Read the model definition and answer for the solid it produces. Units are mm, in the model's axes. A direction names the side the tool comes from. Coordinates: 2 decimals unless noted, no trailing zeros. Write each loop counter-clockwise with the first axis right and the second up, starting at its lowest first coordinate (ties: lowest second). Pieces come first, ordered by that corner, then holes. Notation, with made-up numbers: (82.25, 52.25) -> (141.25, 52.25) arc R19 cw to (141.25, 61.25) -> close; hole circle Ø5 at (-19.5, -16.5). An arc over 180 degrees is marked (long way). Answer as a JSON object with one key per item and string values. Group by question number.
(1) Find section C-C (x = 46). Give the vertices of the cut face in (y, z).
(2) For a pull along X with two mould halves and no side action, classify faces 4 (the face through (98.32, 3.24, 1.48)), 5 (the face through (97.908, -0.601, 1.479)), 6 (the face through (-94.092, -0.601, 1.479)), 7 (the face through (-3, 0, 6)) as +X half, -X half, draft (parallel to the pull), parting line (faces both ways), or undercut.
(3) Flat-ended cylindrical pins translate along their axes: P1, Ø2.5, axis at x = -44.5, y = 0, coming from the +Z side; P2, Ø4, axis at y = 2.5, z = -6, coming from the -X side; P3, Ø10, axis at x = 3.5, z = 6.5, coming from the -Y side; P4, Ø3, axis at y = -2, z = 3.5, coming from the -X side. Find the tip coordinate at first contact, or state that the pin passes through.
(4) Straight lines are drawn through the part: L1, parallel to Z at x = 88, y = 4.25; L2, parallel to Y at x = -96, z = 1.55; L3, parallel to X at y = -1.5, z = 8.5. For each, find the intervals that lie inside material, in ascending order.
(5) Find section A-A (x = 0). Give the vertices of the cut face in (y, z).
(6) Find section B-B (z = -3.5). Give the vertices of the cut face in (x, y), then the cut area to 3 significant figures.
(7) Which of the six approach directions +Z, -Z, +X, -X, +Y, -Y give full straight-line access (tool end or side, diameter ignored) to faces 1 (the face through (-3, 0.1, 11.5)), 2 (the face through (0, 0, -9)), 3 (the face through (-3, 0, -3))?
from build123d import *

# Parameters (mm, degrees)
F0_W        = 200
F0_H        = 9
F1_DEPTH    = 3
F2_R        = 2
F3_DEPTH    = 25
F4_T1_DEPTH = 28
F5_R        = 3
F6_DEPTH    = 9
F8_R        = 1


# Not quite as in the source:
# - a fillet or chamfer that OpenCascade refuses, or shapes differently, is made with other operations: its cross-section is extruded or revolved along the edge and cut away or added


with BuildPart() as f1:
    # F0 (on Top) → F1 (new body)
    with BuildSketch(Plane.XY):
        Rectangle(F0_W, F0_H)
    extrude(amount=F1_DEPTH)

    # F2 (on face) → F3 (cut)
    with BuildSketch(Plane(origin=(0, 0, 0), x_dir=(1, 0, 0), z_dir=(0, 0, -1))):
        with Locations((-96, 0)):
            Circle(F2_R)
        with Locations((96, 0)):
            Circle(F2_R)
    extrude(amount=-F3_DEPTH, mode=Mode.SUBTRACT)

    # F4: fillet of radius 5 on 4 edges, made by hand

    # F4_s2 → F4_t1 (cut)
    with BuildSketch(Plane.XY.offset(-12.5)):
        with BuildLine():
            ThreePointArc((95, 4.5), (98.5355339059, 3.0355339059), (100, -0.5))
            Line((100, -0.5), (100, 4.5))
            Line((100, 4.5), (95, 4.5))
        make_face()
        with BuildLine():
            ThreePointArc((100, 0.5), (98.5355339059, -3.0355339059), (95, -4.5))
            Line((95, -4.5), (100, -4.5))
            Line((100, -4.5), (100, 0.5))
        make_face()
        with BuildLine():
            ThreePointArc((-95, 4.5), (-98.5355339059, 3.0355339059), (-100, -0.5))
            Line((-100, -0.5), (-100, 4.5))
            Line((-100, 4.5), (-95, 4.5))
        make_face()
        with BuildLine():
            ThreePointArc((-100, 0.5), (-98.5355339059, -3.0355339059), (-95, -4.5))
            Line((-95, -4.5), (-100, -4.5))
            Line((-100, -4.5), (-100, 0.5))
        make_face()
    extrude(amount=F4_T1_DEPTH, mode=Mode.SUBTRACT)

    # F5 (on face) → F6 (join)
    with BuildSketch(Plane.XY.offset(3)):
        Circle(F5_R)
    extrude(amount=F6_DEPTH)

    # F8 (on face) → F9 (revolve, cut)
    with BuildSketch(Plane(origin=(0, 0, 0), x_dir=(-1, 0, 0), z_dir=(0, 1, 0))):
        with Locations((-3, 10)):
            Circle(F8_R)
    revolve(axis=Axis((0, 0, 12), (0, 0, 1)), mode=Mode.SUBTRACT)

    # F14: F1 across plane


with BuildPart() as f1_1:
    add(f1.part)
    add(f1.part.mirror(Plane(origin=(95, -4.5, 1.5), x_dir=(-1, 0, 0), z_dir=(0, 0, 1))))


solid = f1_1.part
Results below:
{
 "1": {"outline": "(-4.5, 0) -> (4.5, 0) -> (4.5, 3) -> (-4.5, 3) -> close"},
 "2": {"face 4": "+X half", "face 5": "undercut", "face 6": "undercut", "face 7": "parting line"},
 "3": {"P1": "stops at z = 3", "P2": "stops at x = -2.96", "P3": "stops at y = -4.5", "P4": "stops at x = -99.88"},
 "4": {"L1": "z = 0 to 3", "L2": "y = -4.4 to -2, 2 to 4.4", "L3": "x = -2.6 to 2.6"},
 "5": {"outline": "(-4.5, 0) -> (-3, 0) -> (-3, -6) arc R1 cw to (-3, -8) -> (-3, -9) -> (3, -9) -> (3, -8) arc R1 cw to (3, -6) -> (3, 0) -> (4.5, 0) -> (4.5, 3) -> (3, 3) -> (3, 9) arc R1 cw to (3, 11) -> (3, 12) -> (-3, 12) -> (-3, 11) arc R1 cw to (-3, 9) -> (-3, 3) -> (-4.5, 3) -> close"},
 "6": {"outline": "circle Ø6 at (0, 0)", "area": "28.3 mm2"},
 "7": {"face 1": "+Z", "face 2": "-Z, +X, -X, +Y, -Y", "face 3": "-Z"}
}
